Input: part model. Units: mm. Frame: model coordinates. A direction names the side the tool comes from. Coordinates: 2 decimals unless noted, no trailing zeros. Order: outer loops, then holes, each group sorted by start corner. A loop starts at its lowest first (then second) coordinate and runs counter-clockwise, first axis right, second up. Notation, with made-up numbers: M 24.25,-9 L 50.25,-9 A28 ccw 50.25,29 Z; hole C 21.25,-36 d11. An arc over 180 degrees is marked long. One line per item, written item: value.
```python
from build123d import *

# Parameters (mm, degrees)
PAD_DEPTH       = 7
SKETCH006_W     = 14
SKETCH006_H     = 14
PAD002_DEPTH    = 3
POCKET004_DEPTH = 2
SKETCH008_R     = 0.9
POCKET005_DEPTH = 1.001
FILLET_R        = 1.5


with BuildPart() as clamp_unit:
    # Sketch → Pad (new body, symmetric)
    with BuildSketch(Plane.XZ):
        Polygon((-2.6, 3.8), (4.2, 3.8), (4.2, 0), (2.6, 0), (2.6, 2.6), (-2.6, 2.6), (-2.6, 0), (-4.2, 0), (-4.2, 3.8), align=None)
    extrude(amount=PAD_DEPTH, both=True)


with BuildPart() as wire_holder_single_rounded:
    # Sketch006 → Pad002 (new body)
    with BuildSketch(Plane.XY):
        Rectangle(SKETCH006_W, SKETCH006_H)
    extrude(amount=PAD002_DEPTH)

    # Sketch007 → Pocket004 (cut)
    with BuildSketch(Plane.XY.offset(3)):
        with BuildLine():
            Line((-3, 7), (-3, 4.963869))
            ThreePointArc((-3, 4.963869), (-5.8, 0), (-3, -4.963869))
            Line((-3, -7), (-3, -4.963869))
            Line((3, -7), (-3, -7))
            Line((3, -4.963869), (3, -7))
            ThreePointArc((3, -4.963869), (5.8, 0), (3, 4.963869))
            Line((3, 7), (3, 4.963869))
            Line((-3, 7), (3, 7))
        make_face()
    extrude(amount=-POCKET004_DEPTH, mode=Mode.SUBTRACT)

    # Sketch008 → Pocket005 (cut, through all)
    with BuildSketch(Plane.XY.offset(1)):
        Circle(SKETCH008_R)
    extrude(amount=-POCKET005_DEPTH, mode=Mode.SUBTRACT)


with BuildPart() as wire_holder_single_rounded_1:
    # Clone placement: moved
    add(wire_holder_single_rounded.part.moved(Location((-11.2, 0, 0))))

    # Fusion: union clamp-unit
    add(clamp_unit.part)

    # Fillet
    fillet_edges = [wire_holder_single_rounded_1.edges().sort_by_distance(p)[0] for p in [
        (-18.2, -7, 1.5),
        (-18.2, 7, 1.5),
        (4.2, 7, 1.9),
        (4.2, -7, 1.9),
    ]]
    fillet(fillet_edges, radius=FILLET_R)


solid = wire_holder_single_rounded_1.part
```
(1) Access query for faces 1 (the cylindrical face through (-17.77, -6.55, 1.52)), 2 (the flat face through (-2.6, 0, 1)), 3 (the cylindrical face through (-17, 0, 2)), 4 (the flat face through (-14.2, -6, 2)), 5 (the flat face through (-18, 0, 3)). Directions: +Z, -Z, +X, -X, +Y, -Y. A direction counts if a zero-diameter tool reaches every point of the face in a straight line with its end or side. Return the directions, or none.
Data:
face 1: +Z, -Z, -X, -Y
face 2: -Z, +Y, -Y
face 3: +Z
face 4: +Z, +Y, -Y
face 5: +Z, -X, +Y, -Y
(2) First-contact query: pin 1 (2 mm diameter, centred on x = -16.5, y = 1, fed in from +Z); pin 2 (0.6 mm diameter, centred on y = 6.5, z = 2, fed in from -X); pin 3 (1 mm diameter, centred on y = -6.5, z = 2, fed in from -X). Flat tips, straight axial feed; report the tip coordinate or a pass-through.
Data:
pin 1: stops at z = 3
pin 2: stops at x = -18.03
pin 3: stops at x = -18.11
(3) Cut plane B-B on z = 0.5. Output: boundary loops of the cut face in (x, y), plus the area to 3 significant figures.
Data:
outline: M -18.2,-5.5 A1.5 ccw -16.7,-7 L -2.6,-7 L -2.6,7 L -16.7,7 A1.5 ccw -18.2,5.5 Z; M 2.6,-7 L 2.7,-7 A1.5 ccw 4.2,-5.5 L 4.2,5.5 A1.5 ccw 2.7,7 L 2.6,7 Z; hole C -11.2,0 d1.8
area: 236 mm2
(4) Cut plane D-D on z = 1.9. Output: boundary loops of the cut face in (x, y).
Data:
outline: M -18.2,-5.5 A1.5 ccw -16.7,-7 L -14.2,-7 L -14.2,-4.96 A5.8 cw -14.2,4.96 L -14.2,7 L -16.7,7 A1.5 ccw -18.2,5.5 Z; M -8.2,-7 L -2.6,-7 L -2.6,7 L -8.2,7 L -8.2,4.96 A5.8 cw -8.2,-4.96 Z; M 2.6,-7 L 2.7,-7 A1.5 ccw 4.2,-5.5 L 4.2,5.5 A1.5 ccw 2.7,7 L 2.6,7 Z
(5) Cut plane C-C on y = 0. Output: boundary loops of the cut face in (x, z).
Data:
outline: M -18.2,0 L -12.1,0 L -12.1,1 L -17,1 L -17,3 L -18.2,3 Z; M -10.3,0 L -2.6,0 L -2.6,2.6 L 2.6,2.6 L 2.6,0 L 4.2,0 L 4.2,3.8 L -4.2,3.8 L -4.2,3 L -5.4,3 L -5.4,1 L -10.3,1 Z
(6) Ray query, line 1 (X direction, y = 4.25, z = 1.05); line 2 (Y direction, x = -11.2, z = 0.5); line 3 (X direction, y = 1.5, z = 0.75). Return the intervals inside material, ascending. Write a range as from..to.
Data:
line 1: x = -18.2..-15.15, -7.25..-2.6, 2.6..4.2
line 2: y = -7..-0.9, 0.9..7
line 3: x = -18.2..-2.6, 2.6..4.2
(7) Draft query along X for faces 6 (the cylindrical face through (-12.1, 0, 0.5)), 7 (the cylindrical face through (3.77, 6.55, 1.87)), 8 (the flat face through (-8.2, -6, 2)), 9 (the flat face through (-7, 7, 2)). Return one class per face: released by +X, released by -X, zero draft, split by the parting line, or undercut.
Data:
face 6: undercut
face 7: released by +X
face 8: undercut
face 9: zero draft
(8) Cut plane A-A on x = -11.2. Output: boundary loops of the cut face in (y, z).
Data:
outline: M -7,0 L -0.9,0 L -0.9,1 L -7,1 Z; M 0.9,0 L 7,0 L 7,1 L 0.9,1 Z
